from build123d import *

# Parameters (mm, degrees)
F0_R     = 148.5
F0_R_2   = 8.3312
F1_DEPTH = 20
F2_R     = 146.5
F2_R_2   = 142
F3_DEPTH = 5


# Not quite as in the source:
# - a feature names something its author has since deleted; it is built from what else it names


with BuildPart() as f1:
    # F0 (on Top) → F1 (new body)
    with BuildSketch(Plane.XY):
        Circle(F0_R)
        with Locations((0, 60)):
            Circle(F0_R_2, mode=Mode.SUBTRACT)
    extrude(amount=F1_DEPTH)

    # F2 (on face) → F3 (cut)
    with BuildSketch(Plane.XY):
        Circle(F2_R)
        Circle(F2_R_2, mode=Mode.SUBTRACT)
    extrude(amount=F3_DEPTH, mode=Mode.SUBTRACT)


solid = f1.part
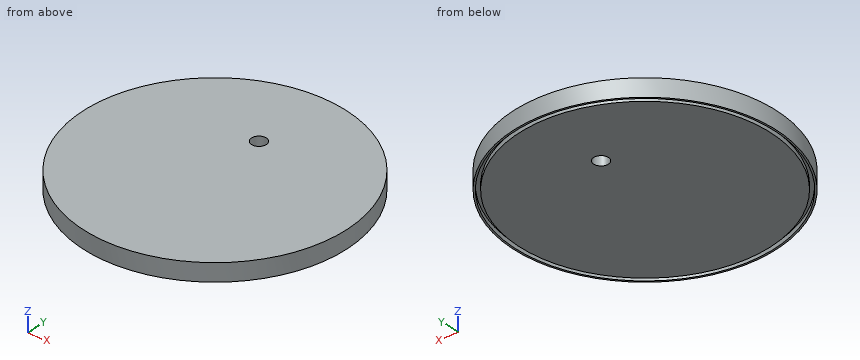
Model file for the job. Use its own axes, mm. Round coordinates to 2 decimals unless told otherwise and drop trailing zeros. Order: outer loops, then holes, each group sorted by start corner. A loop starts at its lowest first (then second) coordinate and runs counter-clockwise, first axis right, second up.
(1) Pin check, flat tips, straight feed: pin 1 (15 mm diameter, centred on x = 0, y = 60, fed in from +Z); pin 2 (1 mm diameter, centred on y = -92, z = 6.5, fed in from +X); pin 3 (2 mm diameter, centred on y = 96, z = 10.5, fed in from -X); pin 4 (1.5 mm diameter, centred on y = 115.5, z = 6, fed in from +X). Stop position of each tip, or through.
(2) Band-saw the part on C-C (z = 8). List the corners of the cut face in (x, y), then the cut area to 3 significant figures.
(3) Band-saw the part on A-A (x = 0). List the corners of the cut face in (y, z).
(4) Band-saw the part on B-B (y = 60). List the corners of the cut face in (x, z).
(5) Band-saw the part on D-D (x = 33). List the corners of the cut face in (y, z).
(6) Drill centre lines: line 1 (Y direction, x = 0, z = 1.15); line 2 (Y direction, x = 0, z = 12); line 3 (Y direction, x = -84.5, z = 2.25). Where is each one in solid material? Low to high.
Verdict:
1. pin 1: passes through
1. pin 2: stops at x = 116.96
1. pin 3: stops at x = -114.14
1. pin 4: stops at x = 94.26
2. outline: circle Ø297 at (0, 0); hole circle Ø16.66 at (0, 60)
2. area: 69,100 mm2
3. outline: (-148.5, 0) - (-146.5, 0) - (-146.5, 5) - (-142, 5) - (-142, 0) - (51.67, 0) - (51.67, 20) - (-148.5, 20) - close; (68.33, 0) - (142, 0) - (142, 5) - (146.5, 5) - (146.5, 0) - (148.5, 0) - (148.5, 20) - (68.33, 20) - close
4. outline: (-135.84, 0) - (-133.65, 0) - (-133.65, 5) - (-128.7, 5) - (-128.7, 0) - (-8.33, 0) - (-8.33, 20) - (-135.84, 20) - close; (8.33, 0) - (128.7, 0) - (128.7, 5) - (133.65, 5) - (133.65, 0) - (135.84, 0) - (135.84, 20) - (8.33, 20) - close
5. outline: (-144.79, 0) - (-142.73, 0) - (-142.73, 5) - (-138.11, 5) - (-138.11, 0) - (138.11, 0) - (138.11, 5) - (142.73, 5) - (142.73, 0) - (144.79, 0) - (144.79, 20) - (-144.79, 20) - close
6. line 1: y = -148.5 to -146.5, -142 to 51.67, 68.33 to 142, 146.5 to 148.5
6. line 2: y = -148.5 to 51.67, 68.33 to 148.5
6. line 3: y = -122.11 to -119.67, -114.12 to 114.12, 119.67 to 122.11
